The model under review builds one solid part; all positions refer to its coordinate system, in mm. Face numbers are marked on the shaded views. A direction names the side the tool comes from. Give positions to 0.01 mm unless a question says otherwise; leave off trailing zeros. Order: outer loops, then holes, each group sorted by start corner. A loop starts at its lowest first (then second) coordinate and runs counter-clockwise, first axis right, second up.
```python
from build123d import *

# Parameters (mm, degrees)
F0_W     = 98
F0_H     = 60
F0_R     = 1.8
F1_DEPTH = 1.64
F2_W     = 98
F2_H     = 40
F3_DEPTH = 9.46
F4_W     = 84
F4_H     = 4
F5_DEPTH = 3
F7_DEPTH = 15


with BuildPart() as f1:
    # F0 (on Top) → F1 (new body)
    with BuildSketch(Plane.XY):
        Rectangle(F0_W, F0_H)
        with Locations((-46.5, -27.5)):
            Circle(F0_R, mode=Mode.SUBTRACT)
        with Locations((46.5, -27.5)):
            Circle(F0_R, mode=Mode.SUBTRACT)
        with Locations((-46.5, 27.5)):
            Circle(F0_R, mode=Mode.SUBTRACT)
        with Locations((46.5, 27.5)):
            Circle(F0_R, mode=Mode.SUBTRACT)
    extrude(amount=F1_DEPTH)

    # F2 (on face) → F3 (join)
    with BuildSketch(Plane.XY.offset(1.64)):
        Rectangle(F2_W, F2_H)
    extrude(amount=F3_DEPTH)

    # F4 (on face) → F5 (join)
    with BuildSketch(Plane.XY.offset(1.64)):
        with Locations((0, 28)):
            Rectangle(F4_W, F4_H)
    extrude(amount=F5_DEPTH)

    # F6 (on face) → F7 (join)
    with BuildSketch(Plane(origin=(0, 0, 0), x_dir=(1, 0, 0), z_dir=(0, 0, -1))):
        Polygon((11, -8), (-49, -8), (-49, -25), (-44, -25), (-44, -30), (11, -30), align=None)
    extrude(amount=F7_DEPTH)


solid = f1.part
```
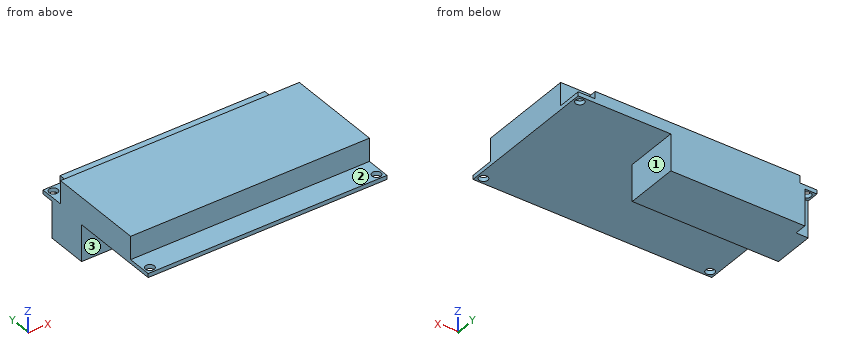
Item 1: For the marked faces 1, 2 and 3, list the 3-axis set-ups (+Z, -Z, +X, -X, +Y, -Y) from which the entire face can be reached by the end or side of a thin tool; tool diameter is ignored.
Values found:
face 1: -Z, +X, +Y, -Y
face 2: +Z, +X, -X, -Y
face 3: -Z, +X, -X, -Y
Item 2: For line 1 (Y direction, x = 46.5, z = 1.2); line 2 (Y direction, x = -27.5, z = 3.75); line 3 (Z direction, x = -17.5, y = -24), list the stretches that pass through material, from the lowest coordinate up.
Values found:
line 1: y = -30 to -29.3, -25.7 to 25.7, 29.3 to 30
line 2: y = -20 to 20, 26 to 30
line 3: z = 0 to 1.64
Item 3: Take a section at A-A (y = -27.5). Give the boundary of the cut face in (x, z).
Values found:
outline: (-49, 0) - (-48.3, 0) - (-48.3, 1.64) - (-49, 1.64) - close; (-44.7, 0) - (44.7, 0) - (44.7, 1.64) - (-44.7, 1.64) - close; (48.3, 0) - (49, 0) - (49, 1.64) - (48.3, 1.64) - close
Item 4: Take a section at C-C (y = 27.5). Give the boundary of the cut face in (x, z).
Values found:
outline: (-49, 0) - (-48.3, 0) - (-48.3, 1.64) - (-49, 1.64) - close; (-44.7, 0) - (-44, 0) - (-44, -15) - (11, -15) - (11, 0) - (44.7, 0) - (44.7, 1.64) - (42, 1.64) - (42, 4.64) - (-42, 4.64) - (-42, 1.64) - (-44.7, 1.64) - close; (48.3, 0) - (49, 0) - (49, 1.64) - (48.3, 1.64) - close
Item 5: Clearance check with flat-ended pins moving along their axes: pin 1 Ø3 at (x, y) = (15.5, -21.5) entering from -Z; pin 2 Ø1.2 at (x, y) = (-17.5, 27.5) entering from +Z; pin 3 Ø3 at (x, y) = (-19, -25) entering from +Z; pin 4 Ø2 at (x, y) = (-46.5, -27.5) entering from +Z. State where each tip first meets the part, or that it passes through.
Values found:
pin 1: stops at z = 0
pin 2: stops at z = 4.64
pin 3: stops at z = 1.64
pin 4: passes through
Item 6: Take a section at B-B (x = -46.5). Give the boundary of the cut face in (y, z).
Values found:
outline: (-30, 0) - (-29.3, 0) - (-29.3, 1.64) - (-30, 1.64) - close; (-25.7, 0) - (8, 0) - (8, -15) - (25, -15) - (25, 0) - (25.7, 0) - (25.7, 1.64) - (20, 1.64) - (20, 11.1) - (-20, 11.1) - (-20, 1.64) - (-25.7, 1.64) - close; (29.3, 0) - (30, 0) - (30, 1.64) - (29.3, 1.64) - close
Item 7: Take a section at D-D (z = 7.75). Give the boundary of the cut face in (x, y), and give its area (3 significant figures).
Values found:
outline: (-49, -20) - (49, -20) - (49, 20) - (-49, 20) - close
area: 3,920 mm2
